from build123d import *

# Parameters (mm, degrees)
EXTRUDE_2_DEPTH = 7
SKETCH_4_R      = 8.164253287
EXTRUDE_3_DEPTH = 7


with BuildPart() as part:
    # 草图2 → 凸台-拉伸2 (new body)
    with BuildSketch(Plane(origin=(0, 0, 0), x_dir=(1, 0, 0), z_dir=(0, 1, 0))):
        Polygon((0, 230), (0, 160), (-40, 160), (-40, 70), (0, 70), (0, 0), (70, 0), (70, 70), (110, 70), (110, 160), (70, 160), (70, 230), align=None)
    extrude(amount=EXTRUDE_2_DEPTH)

    # 草图4 → 凸台-拉伸3 (add)
    with BuildSketch(Plane(origin=(0, 7, 0), x_dir=(1, 0, 0), z_dir=(0, 1, 0))):
        with Locations(Location((35, 8.164253287, 0), (0, 0, 270))):
            Circle(SKETCH_4_R)
    extrude(amount=EXTRUDE_3_DEPTH)


solid = part.part
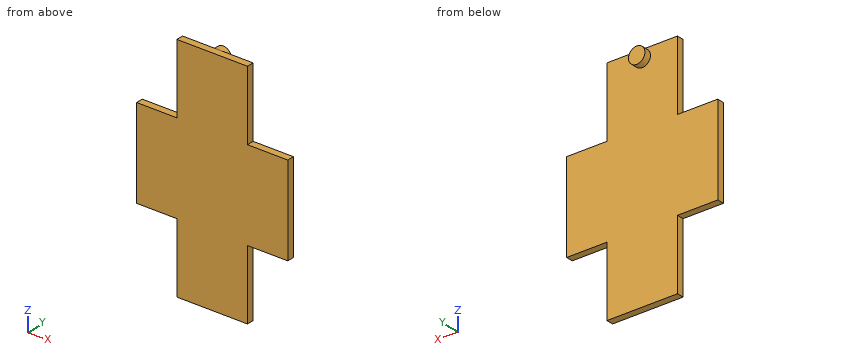
The listing builds one solid part. Answer for the finished solid, in the listing's coordinates (mm). Round coordinates to 2 decimals unless told otherwise and drop trailing zeros. Write each loop counter-clockwise with the first axis right and the second up, starting at its lowest first coordinate (ties: lowest second). Pieces come first, ordered by that corner, then holes. Notation, with made-up numbers: (34, -35.5) - (56, -35.5) arc R17 cw to (56, -24.5) - close; hole circle Ø10 at (43, 75.5). An arc over 180 degrees is marked (long way). Use a Markdown table: item, result. Add a question column.
1. Consider line 1 (X direction, y = 5.75, z = -201); line 2 (Z direction, x = 96, y = 1.75); line 3 (Y direction, x = 44.5, z = -33.5). Determine where each line is inside the solid, lowest interval first.
2. The part is cut by section C-C (z = -46). Write down the section's boundary in (x, y).
3. The part is cut by section B-B (x = 75.5). Write down the section's boundary in (y, z), and give its area (3 significant figures).
4. The part is cut by section A-A (y = 2.25). Write down the section's boundary in (x, z), and give its area (3 significant figures).
5. Flat-ended cylindrical pins translate along their axes: P1, Ø1.5, axis at x = -24, y = 6.5, coming from the +Z side; P2, Ø3.5, axis at y = 5, z = -17.5, coming from the -X side; P3, Ø7.5, axis at y = 4, z = -22, coming from the +X side; P4, Ø3, axis at y = 10, z = -156, coming from the -X side. Find the tip coordinate at first contact, or state that the pin passes through.
Reported:
| question | item | result |
|---|---|---|
| 1 | line 1 | 0 to 70 |
| 1 | line 2 | -160 to -70 |
| 1 | line 3 | 0 to 7 |
| 2 | outline | (0, 0) - (70, 0) - (70, 7) - (0, 7) - close |
| 3 | outline | (0, -160) - (7, -160) - (7, -70) - (0, -70) - close |
| 3 | area | 630 mm^2 |
| 4 | outline | (-40, -160) - (0, -160) - (0, -230) - (70, -230) - (70, -160) - (110, -160) - (110, -70) - (70, -70) - (70, 0) - (0, 0) - (0, -70) - (-40, -70) - close |
| 4 | area | 23,300 mm^2 |
| 5 | P1 | z = -70 |
| 5 | P2 | x = 0 |
| 5 | P3 | x = 70 |
| 5 | P4 | through |
